For this review, take the finished solid that the model builds, in its own axes (mm). Face numbers are marked on the shaded views. Round coordinates to 2 decimals unless told otherwise and drop trailing zeros. Write each loop counter-clockwise with the first axis right and the second up, starting at its lowest first coordinate (ties: lowest second). Pieces come first, ordered by that corner, then holes. Notation, with made-up numbers: M 16.5,34 L 41.5,34 A19 cw 41.5,56 Z; hole C 27,25 d7. An arc over 180 degrees is marked long. Answer in a Markdown table with one row per item.
```python
from build123d import *

# Parameters (mm, degrees)
SKETCH1_W                = 8
SKETCH1_H                = 47.5
BOSS_EXTRUDE1_DEPTH      = 5
BOSS_EXTRUDE2_DEPTH      = 1.9
BOSS_EXTRUDE2_DEPTH_BACK = 10.4
SKETCH2_R                = 1.5
FILLET1_R                = 2.5


with BuildPart() as part:
    # Sketch1 → Boss-Extrude1 (new body)
    with BuildSketch(Plane(origin=(0, 0, 0), x_dir=(1, 0, 0), z_dir=(0, 1, 0))):
        with Locations((4, 23.75)):
            Rectangle(SKETCH1_W, SKETCH1_H)
    extrude(amount=BOSS_EXTRUDE1_DEPTH)

    # Sketch2 → Boss-Extrude2 (add, two sides: drawn at the far end of the back side and taken through both)
    with BuildSketch(Plane(origin=(8, 0, 0), x_dir=(0, 0, -1), z_dir=(1, 0, 0)).offset(-BOSS_EXTRUDE2_DEPTH_BACK)):
        with Locations((2.5, 2.5)):
            Circle(SKETCH2_R)
        with Locations((45, 2.5)):
            Circle(SKETCH2_R)
    extrude(amount=BOSS_EXTRUDE2_DEPTH + BOSS_EXTRUDE2_DEPTH_BACK)

    # Fillet1
    fillet1_edges = [part.edges().sort_by_distance(p)[0] for p in [
        (4, 0, -47.5),
        (4, 5, -47.5),
        (4, 0, 0),
        (4, 5, 0),
    ]]
    fillet(fillet1_edges, radius=FILLET1_R - 0.0001)  # a hair under: the kernel refuses the full size


solid = part.part
```
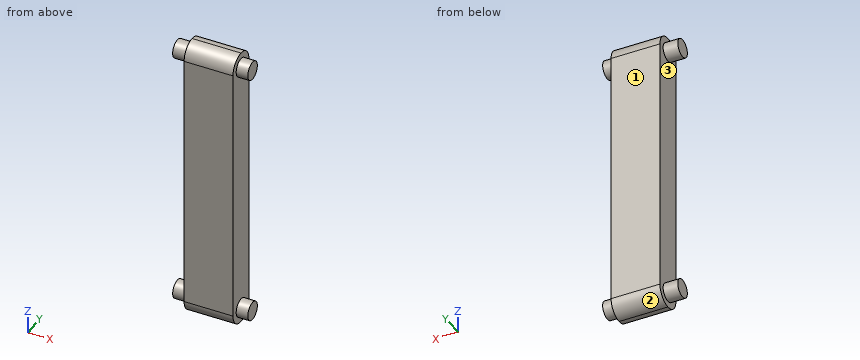
Q1. Take a section at C-C (z = -21). State the section outline as (x, y) points.
Found:
| item | result |
|---|---|
| outline | M 0,0 L 8,0 L 8,5 L 0,5 Z |
Q2. For probe 1 along X at (y, z) = (4.05, -28); probe 2 along Z at (x, y) = (1.25, 2.4); probe 3 along Z at (x, y) = (3, 4.5), list the stretches that pass through material, from the lowest coordinate up.
Found:
| item | result |
|---|---|
| probe 1 | 0 to 8 |
| probe 2 | -47.5 to 0 |
| probe 3 | -46.5 to -1 |
Q3. Take a section at B-B (y = 1.75). State the section outline as (x, z) points.
Found:
| item | result |
|---|---|
| outline | M -2.4,-46.3 L 0,-46.3 L 0,-47.38 L 8,-47.38 L 8,-46.3 L 9.9,-46.3 L 9.9,-43.7 L 8,-43.7 L 8,-3.8 L 9.9,-3.8 L 9.9,-1.2 L 8,-1.2 L 8,-0.12 L 0,-0.12 L 0,-1.2 L -2.4,-1.2 L -2.4,-3.8 L 0,-3.8 L 0,-43.7 L -2.4,-43.7 Z |
Q4. Insertion check: P1, Ø1.5, axis at y = 3.5, z = -13, coming from the -X side; P2, Ø1.5, axis at y = 1.5, z = -25.5, coming from the +X side. Each pin has a flat end and moves straight along its axis. Give the tip position at first contact, or say it passes through.
Found:
| item | result |
|---|---|
| P1 | x = 0 |
| P2 | x = 8 |
Q5. Mouldability with a two-part tool opening along Z and no side actions: class the marked faces 1, 2 and 3 as +Z half, -Z half, draft (parallel to the pull), parting line (faces both ways), or undercut.
Found:
| item | result |
|---|---|
| face 1 | draft |
| face 2 | -Z half |
| face 3 | undercut |
